Job drawing, mm, ordinate dimensions from the low corner. One solid piece. Give positions to 0.01 mm unless a question says otherwise; leave off trailing zeros. Write each loop counter-clockwise with the first axis right and the second up, starting at its lowest first coordinate (ties: lowest second). Pieces come first, ordered by that corner, then holes. Notation, with made-up numbers: (81.25, 20.25) -> (101.25, 20.25) arc R3 ccw to (101.25, 25.25) -> close; hole circle Ø10 at (86.25, -31.75). An arc over 180 degrees is marked (long way). One line per question, with ' | ' between items. Start each with the question number.
(1) Band-saw the part on A-A, the plane x = 57.55. Give the cut face in (y, z).
(2) Drill centre lines: probe 1 along Z at (x, y) = (55.5, 6.25); probe 2 along Z at (x, y) = (57.55, 16); probe 3 along X at (y, z) = (13.25, 78). Where is each one in solid material? Low to high. Write a range as from..to.
(3) Band-saw the part on B-B, the plane y = 8.75. Give the cut face in (x, z).
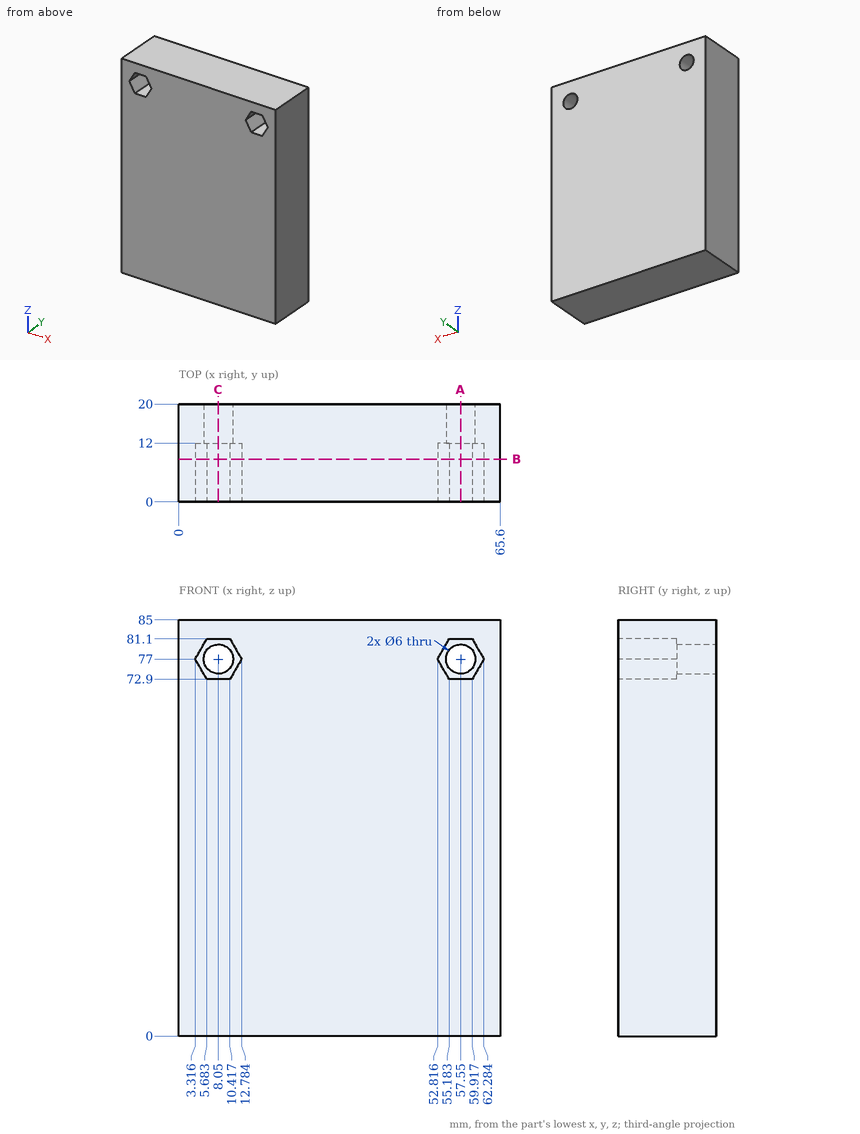
Results:
1) outline: (0, 0) -> (20, 0) -> (20, 74) -> (12, 74) -> (12, 72.9) -> (0, 72.9) -> close; (0, 81.1) -> (12, 81.1) -> (12, 80) -> (20, 80) -> (20, 85) -> (0, 85) -> close
2) probe 1: z = 0..72.9, 81.1..85 | probe 2: z = 0..74, 80..85 | probe 3: x = 0..5.22, 10.88..54.72, 60.38..65.6
3) outline: (0, 0) -> (65.6, 0) -> (65.6, 85) -> (0, 85) -> close; hole (3.32, 77) -> (5.68, 72.9) -> (10.42, 72.9) -> (12.78, 77) -> (10.42, 81.1) -> (5.68, 81.1) -> close; hole (52.82, 77) -> (55.18, 72.9) -> (59.92, 72.9) -> (62.28, 77) -> (59.92, 81.1) -> (55.18, 81.1) -> close
